The model under review builds one solid part; all positions refer to its coordinate system, in mm. Give positions to 0.01 mm unless a question says otherwise; leave off trailing zeros. Loops run counter-clockwise (first coordinate to the right, second up) from the corner with the lowest first, then second, coordinate; pieces in that order, holes last. Notation, with made-up numbers: M -15,0.5 L 42,0.5 A15 ccw 42,18.5 Z; hole C -19,40.25 d9. An arc over 180 degrees is marked long. Put each result on its own line as item: value. Start each with the question number.
```python
from build123d import *

# Parameters (mm, degrees)
SKETCH1_R           = 2.413
SKETCH1_R_2         = 14.2875
SKETCH1_R_3         = 12.7
BOSS_EXTRUDE1_DEPTH = 6.35
SKETCH2_R           = 2.413
CUT_EXTRUDE1_DEPTH  = 104.930431183
SKETCH3_R           = 2.413
CUT_EXTRUDE2_DEPTH  = 104.930431183
FILLET1_R           = 3.175
CUT_EXTRUDE4_DEPTH  = 104.930431183
FILLET2_R           = 3.175


with BuildPart() as part:
    # Sketch1 → Boss-Extrude1 (new body)
    with BuildSketch(Plane.XY):
        with BuildLine():
            Line((-36.83, -38.1), (36.83, -38.1))
            Line((36.83, -38.1), (36.83, 0))
            Line((36.83, 0), (36.83, 13.898506919))
            ThreePointArc((36.83, 13.898506919), (37.741105518, 16.124581216), (39.95151608, 17.07305641))
            ThreePointArc((39.95151608, 17.07305641), (69.442535879, 47.318867003), (39.4462, 77.0636))
            Line((39.4462, 77.0636), (-39.4462, 77.0636))
            ThreePointArc((-39.4462, 77.0636), (-69.442535879, 47.318867003), (-39.95151608, 17.07305641))
            ThreePointArc((-39.95151608, 17.07305641), (-37.741105518, 16.124581216), (-36.83, 13.898506919))
            Line((-36.83, 13.898506919), (-36.83, 0))
            Line((-36.83, 0), (-36.83, -38.1))
        make_face()
        with Locations((-30.48, -31.75)):
            Circle(SKETCH1_R, mode=Mode.SUBTRACT)
        with Locations((0, -25.4)):
            Circle(SKETCH1_R, mode=Mode.SUBTRACT)
        with Locations((30.48, -31.75)):
            Circle(SKETCH1_R, mode=Mode.SUBTRACT)
        Circle(SKETCH1_R_2, mode=Mode.SUBTRACT)
        with Locations((-39.4462, 47.0662)):
            Circle(SKETCH1_R_3, mode=Mode.SUBTRACT)
        with Locations((0, 47.0662)):
            Circle(SKETCH1_R_2, mode=Mode.SUBTRACT)
        with Locations((39.4462, 47.0662)):
            Circle(SKETCH1_R_3, mode=Mode.SUBTRACT)
        with Locations((52.1462, 69.063245256)):
            Circle(SKETCH1_R, mode=Mode.SUBTRACT)
    extrude(amount=BOSS_EXTRUDE1_DEPTH)

    # Sketch2 → Cut-Extrude1 (cut, through all)
    with BuildSketch(Plane.XY.offset(6.35)):
        with Locations((-25.4, 0)):
            Circle(SKETCH2_R)
        with Locations((25.4, 0)):
            Circle(SKETCH2_R)
    extrude(amount=-CUT_EXTRUDE1_DEPTH, mode=Mode.SUBTRACT)

    # Sketch3 → Cut-Extrude2 (cut, through all)
    with BuildSketch(Plane.XY.offset(6.35)):
        with Locations((-26.7462, 25.069154744)):
            Circle(SKETCH3_R)
        with Locations((-52.1462, 25.069154744)):
            Circle(SKETCH3_R)
        with Locations((-64.8462, 47.0662)):
            Circle(SKETCH3_R)
        with Locations((-52.1462, 69.063245256)):
            Circle(SKETCH3_R)
        with Locations((-26.7462, 69.063245256)):
            Circle(SKETCH3_R)
        with Locations((26.7462, 25.069154744)):
            Circle(SKETCH3_R)
        with Locations((52.1462, 25.069154744)):
            Circle(SKETCH3_R)
        with Locations((52.1462, 69.063245256)):
            Circle(SKETCH3_R)
        with Locations((64.8462, 47.0662)):
            Circle(SKETCH3_R)
        with Locations((26.7462, 69.063245256)):
            Circle(SKETCH3_R)
    extrude(amount=-CUT_EXTRUDE2_DEPTH, mode=Mode.SUBTRACT)

    # Fillet1
    fillet1_edges = [part.edges().sort_by_distance(p)[0] for p in [
        (36.83, -38.1, 3.175),
        (-36.83, -38.1, 3.175),
    ]]
    fillet(fillet1_edges, radius=FILLET1_R)

    # Sketch4 → Cut-Extrude4 (cut, through all)
    with BuildSketch(Plane.XY.offset(6.35)):
        with BuildLine():
            Line((-20.280551981, 27.712187223), (-9.984322179, 18.061553557))
            ThreePointArc((-9.984322179, 18.061553557), (0, 20.6375), (9.984322179, 18.061553557))
            Line((9.984322179, 18.061553557), (20.280551981, 27.712187223))
            ThreePointArc((20.280551981, 27.712187223), (23.31373077, 31.152606065), (27.826871421, 31.970051372))
            ThreePointArc((27.826871421, 31.970051372), (22.865552696, 37.686187475), (20.521705522, 44.883080962))
            ThreePointArc((20.521705522, 44.883080962), (0, 26.4287), (-20.521705522, 44.883080962))
            ThreePointArc((-20.521705522, 44.883080962), (-22.865552696, 37.686187475), (-27.826871421, 31.970051372))
            ThreePointArc((-27.826871421, 31.970051372), (-23.31373077, 31.152606065), (-20.280551981, 27.712187223))
        make_face()
        with BuildLine():
            ThreePointArc((20.123546875, -4.577036969), (15.228507825, -13.928350788), (6.35, -19.636290542))
            Line((6.35, -19.636290542), (6.35, -31.75))
            Line((6.35, -31.75), (23.495, -31.75))
            ThreePointArc((23.495, -31.75), (25.540859133, -26.810859133), (30.48, -24.765))
            Line((30.48, -24.765), (30.48, -4.794144866))
            ThreePointArc((30.48, -4.794144866), (25.253601853, -6.983465657), (20.123546875, -4.577036969))
        make_face()
        with BuildLine():
            Line((-6.35, -31.75), (-6.35, -19.636290542))
            ThreePointArc((-6.35, -19.636290542), (-15.228507825, -13.928350788), (-20.123546875, -4.577036969))
            ThreePointArc((-20.123546875, -4.577036969), (-25.253601853, -6.983465657), (-30.48, -4.794144866))
            Line((-30.48, -4.794144866), (-30.48, -24.765))
            ThreePointArc((-30.48, -24.765), (-25.540859133, -26.810859133), (-23.495, -31.75))
            Line((-23.495, -31.75), (-6.35, -31.75))
        make_face()
    extrude(amount=-CUT_EXTRUDE4_DEPTH, mode=Mode.SUBTRACT)

    # Fillet2
    fillet2_edges = [part.edges().sort_by_distance(p)[0] for p in [
        (-27.826871421, 31.970051372, 3.175),
        (-20.521705522, 44.883080962, 3.175),
        (20.521705522, 44.883080962, 3.175),
        (27.826871421, 31.970051372, 3.175),
        (20.280551981, 27.712187223, 3.175),
        (9.984322179, 18.061553557, 3.175),
        (-9.984322179, 18.061553557, 3.175),
        (-20.280551981, 27.712187223, 3.175),
        (20.123546875, -4.577036969, 3.175),
        (30.48, -4.794144866, 3.175),
        (30.48, -24.765, 3.175),
        (23.495, -31.75, 3.175),
        (6.35, -31.75, 3.175),
        (6.35, -19.636290542, 3.175),
        (-30.48, -4.794144866, 3.175),
        (-20.123546875, -4.577036969, 3.175),
        (-6.35, -19.636290542, 3.175),
        (-6.35, -31.75, 3.175),
        (-23.495, -31.75, 3.175),
        (-30.48, -24.765, 3.175),
    ]]
    fillet(fillet2_edges, radius=FILLET2_R)


solid = part.part
```
Item 1: To check wall thickness, follow L1, parallel to Y at x = 0, z = 1.5; L2, parallel to X at y = 57.5, z = 2.25; L3, parallel to X at y = 52.5, z = 3. State the ranges of each line that lie inside material, in increasing order. Write a range as [from, to].
Item 2: Consider section D-D, the plane z = 4. Give the number of separate pieces and of enclosed holes in the cut face, plus the area to 3 significant figures.
Item 3: Clearance check with a flat-ended pin moving along its axis: pin 1 Ø1.5 at (x, z) = (48, 2.5) entering from -Y. State where the tip first meets the part, or that it passes through.
Item 4: Draft analysis for pull direction Y (two halves, no side actions). For faces 1 (the cylindrical face through (29.36, -7.56, 3.13)), 2 (the flat face through (36.83, -11, 3)), 3 (the flat face through (1, 77.064, 3)), state which applies: +Y half, -Y half, draft (parallel to the pull), parting line (faces both ways), or undercut.
Item 5: Consider section C-C, the plane y = 52. Write out the cut boundary in (x, z).
Item 6: Consider section B-B, the plane x = 0. Write out the cut boundary in (y, z), plus the area to 3 significant figures.
Item 7: Consider section A-A, the plane y = 0. Write out the cut boundary in (x, z), plus the area to 3 significant figures.
Report:
1. L1: [-38.1, -27.81], [-22.99, -14.29], [14.29, 20.64], [26.43, 32.78], [61.35, 77.06]
1. L2: [-67.57, -46.69], [-32.21, -9.76], [9.76, 32.21], [46.69, 67.57]
1. L3: [-68.95, -50.93], [-27.97, -13.21], [13.21, 27.97], [50.93, 68.95]
2. separate pieces: 1
2. enclosed holes: 22
2. area: 7,740 mm²
3. pin 1: y = 18.1
4. face 1: undercut
4. face 2: draft
4. face 3: +Y half
5. outline: M -69.04,0 L -51.15,0 L -51.15,6.35 L -69.04,6.35 Z; M -27.74,0 L -13.41,0 L -13.41,6.35 L -27.74,6.35 Z; M 13.41,0 L 27.74,0 L 27.74,6.35 L 13.41,6.35 Z; M 51.15,0 L 69.04,0 L 69.04,6.35 L 51.15,6.35 Z
6. outline: M -38.1,0 L -27.81,0 L -27.81,6.35 L -38.1,6.35 Z; M -22.99,0 L -14.29,0 L -14.29,6.35 L -22.99,6.35 Z; M 14.29,0 L 20.64,0 L 20.64,6.35 L 14.29,6.35 Z; M 26.43,0 L 32.78,0 L 32.78,6.35 L 26.43,6.35 Z; M 61.35,0 L 77.06,0 L 77.06,6.35 L 61.35,6.35 Z
6. area: 301 mm²
7. outline: M -36.83,0 L -27.81,0 L -27.81,6.35 L -36.83,6.35 Z; M -22.99,0 L -14.29,0 L -14.29,6.35 L -22.99,6.35 Z; M 14.29,0 L 22.99,0 L 22.99,6.35 L 14.29,6.35 Z; M 27.81,0 L 36.83,0 L 36.83,6.35 L 27.81,6.35 Z
7. area: 225 mm²
